Autodesk Fusion 360 part; units mm, degrees
sketch "Sketch1" plane through (0, 0, 0) normal (1, 0, 0) x (0, 1, 0)
  line L0 (0, 0) -> (31.75, 0)
  line L1 (31.75, 0) -> (31.75, -19.05)
  line L2 (31.75, -19.05) -> (0, -19.05)
  line L3 (0, -19.05) -> (0, 0)
  dimension "d1" = 31.75
  dimension "d2" = 19.05
extrude "Extrude1" add sketch "Sketch1" along normal blind 6.35
sketch "Sketch2" plane through (6.35, 0, 0) normal (1, 0, 0) x (0, 1, 0)
  line L0 (0, -19.05) -> (31.75, -19.05)
  line L1 (31.75, -19.05) -> (31.75, 0)
  line L2 (31.75, 0) -> (0, 0)
  line L3 (0, 0) -> (0, -19.05)
sketch "Sketch3" plane through (6.35, 15.875, -9.525) normal (1, 0, 0) x (0, 1, 0)
  line L0 (15.5884, -0.1633) -> (9.2384, -0.1633)
  line L1 (-15.8946, -0.0015) -> (-3.1946, -0.0015)
  circle A0 centre (-3.1946, -0.0015) radius 4.7625
  dimension "d9" = 6.35
  dimension "d10" = 12.7
  dimension "d11" = 9.525
hole "Hole3" at (6.35, 12.6804, -9.5265) direction (-1, 0, 0) diameter 9.525 depth 50.8 tip angle 118
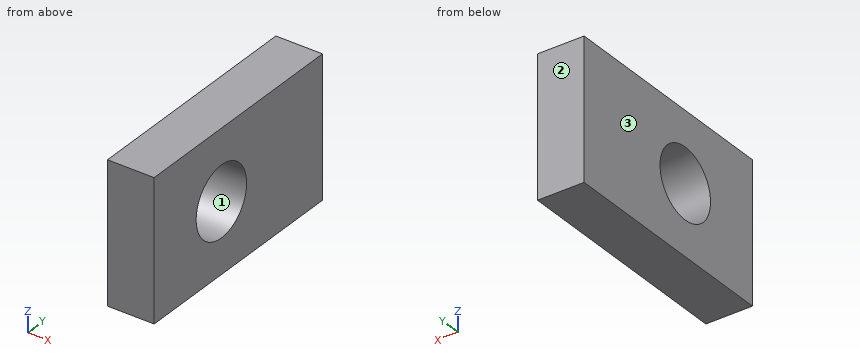
CAD build for the part. Positions are in the model's coordinates, mm. Face numbers are marked on the shaded views. Round coordinates to 2 decimals unless told otherwise and drop trailing zeros. Order: outer loops, then holes, each group sorted by start corner. A loop starts at its lowest first (then second) coordinate and runs counter-clockwise, first axis right, second up.
Q1. Two-plate mould, pull along Y, no slides. Class the marked faces 1, 2 and 3: pulls with the +Y half, pulls with the -Y half, needs draft (parallel to the pull), parting line crosses it, or undercut.
Q2. Slice it at A-A (z = -5.75). Write the cut outline in (x, y).
Q3. Wall check: L1, parallel to Y at x = 5.75, z = -9.75; L2, parallel to Z at x = 2.5, y = 13; L3, parallel to Y at x = 5.5, z = -11.75. Give the ranges that are in metal, low to high.
Q4. Slice it at B-B (y = 15). Write the cut outline in (x, z).
Q5. Drop a flat-ended pin along its axis: pin 1 (1.5 mm diameter, centred on x = 1.5, y = 17, fed in from +Z). Give the stop position or say it passes through.
Results below:
1. face 1: undercut
1. face 2: pulls with the +Y half
1. face 3: needs draft
2. outline: (0, 0) - (6.35, 0) - (6.35, 9.78) - (0, 9.78) - close; (0, 15.58) - (6.35, 15.58) - (6.35, 31.75) - (0, 31.75) - close
3. L1: y = 0 to 7.92, 17.44 to 31.75
3. L2: z = -19.05 to -14.28, -4.77 to 0
3. L3: y = 0 to 8.47, 16.89 to 31.75
4. outline: (0, -19.05) - (6.35, -19.05) - (6.35, -13.69) - (0, -13.69) - close; (0, -5.37) - (6.35, -5.37) - (6.35, 0) - (0, 0) - close
5. pin 1: stops at z = 0
